```python
from build123d import *

# Parameters (mm, degrees)
STOCK_BATTERY_BASE_1_DEPTH   = 7.5
STOCK_BATTERY_BASE_1_2_DEPTH = 4.5
BOSS_EXTRUDE1_DEPTH          = 7.5
CUT_EXTRUDE1_DEPTH           = 7.5


# Read off the part's stored shape, not the designer's step: Stock-battery base-1
with BuildPart() as part:
    # Stock-battery base-1 outline → Stock-battery base-1 (new body)
    with BuildSketch(Plane.XY):
        with BuildLine():
            Line((32.459100066, 42.420690995), (16.459100066, 43.22938712))
            Line((16.459100066, 43.22938712), (16.459100066, -58.832087736))
            Line((16.459100066, -58.832087736), (113.496599029, -53.92747215))
            add(Edge.make_bspline(
                [(113.496599029, -53.92747215), (114.973875685, -53.76034768), (116.389465073, -53.408303088), (118.438931288, -52.658652366), (119.109837198, -52.372048444), (120.430638868, -51.735858399), (121.082915856, -51.384782434), (122.988929436, -50.267489711), (124.197203446, -49.437169981), (126.541735842, -47.677906536), (127.677620036, -46.748450374), (128.850515141, -45.74891878), (128.904828159, -45.702543351), (128.959100066, -45.656116492)],
                knots=[0, 0, 0, 0, 0.125, 0.125, 0.1875, 0.1875, 0.25, 0.25, 0.375, 0.375, 0.5, 0.5, 0.506074438, 0.506074438, 0.506074438, 0.506074438], degree=3))
            Line((128.959100066, -45.656116492), (133.959100066, -45.656116492))
            Line((133.959100066, -45.656116492), (133.959100066, 33.628624999))
            Line((133.959100066, 33.628624999), (128.959100066, 33.628624999))
            add(Edge.make_bspline(
                [(128.959100066, 33.628624999), (128.913387154, 33.667730585), (127.751192536, 34.660386778), (126.568806099, 35.629041088), (124.805320754, 36.953884089), (124.207009004, 37.38378621), (122.992052543, 38.206145046), (122.374602128, 38.599251589), (120.484333172, 39.709851881), (119.174169326, 40.359663675), (117.093195419, 41.124643977), (116.387101294, 41.341482025), (114.957490187, 41.687263925), (114.232477088, 41.816732683), (113.496599029, 41.899982649)],
                knots=[0.494878569, 0.494878569, 0.494878569, 0.494878569, 0.5, 0.625, 0.625, 0.6875, 0.6875, 0.75, 0.75, 0.875, 0.875, 0.9375, 0.9375, 1, 1, 1, 1], degree=3))
            Line((113.496599029, 41.899982649), (32.459100066, 45.99590211))
            Line((32.459100066, 45.99590211), (32.459100066, 42.420690995))
        make_face()
        Polygon((112.616329261, 31.931709487), (112.616012614, -43.959214992), (98.959100066, -44.649483258), (98.959100066, 32.621993758), align=None, mode=Mode.SUBTRACT)
    extrude(amount=STOCK_BATTERY_BASE_1_DEPTH)

    # Stock-battery base-1 2 outline → Stock-battery base-1 2 (add)
    with BuildSketch(Plane.XY):
        Polygon((32.459100066, 45.99590211), (16.459100066, 46.804598235), (16.459100066, 43.22938712), (32.459100066, 42.420690995), align=None)
    extrude(amount=STOCK_BATTERY_BASE_1_2_DEPTH)

    # Sketch1 → Boss-Extrude1 (add)
    with BuildSketch(Plane.ZY.offset(-16.459100066)):
        Polygon((0, 46.804598235), (0, -58.832087736), (7.5, -58.832087736), (7.5, 43.22938712), (4.5, 43.22938712), (4.5, 46.804598235), align=None)
    extrude(amount=BOSS_EXTRUDE1_DEPTH)

    # Sketch2 → Cut-Extrude1 (cut)
    with BuildSketch(Plane.ZY.offset(-8.959100066)):
        Polygon((2.7, 41.42938712), (1.8, 41.42938712), (1.8, -57.032087736), (5.7, -57.032087736), (5.7, 41.42938712), align=None)
    extrude(amount=-CUT_EXTRUDE1_DEPTH, mode=Mode.SUBTRACT)


solid = part.part
```
CAD build for the part. Positions are in the model's coordinates, mm. A direction names the side the tool comes from. Round coordinates to 2 decimals unless told otherwise and drop trailing zeros. Write each loop counter-clockwise with the first axis right and the second up, starting at its lowest first coordinate (ties: lowest second). Pieces come first, ordered by that corner, then holes. Notation, with made-up numbers: (33, -4.5) - (53, -4.5) arc R25 ccw to (53, 25.5) - close; hole circle Ø7 at (6, 46.5). An arc over 180 degrees is marked (long way). Return JSON: item names as keys, results as strings. Group by question number.
Item 1: Mould opens along X. For faces 4 (the face through (131, -45.656, 4)), 5 (the face through (105.69, 32.28, 3.7)), 6 (the face through (16.459, -7, 4)) say: +X half, -X half, draft (parallel to the pull), parting line (faces both ways), or undercut.
Item 2: 3-axis set-ups, long thin cutter, end or side, ignore diameter. For faces 1 (the face through (13, -8, 5.7)), 2 (the face through (131, 33.629, 4)), 3 (the face through (13, 43.229, 6)): which of +Z, -Z, +X, -X, +Y, -Y reach the whole face in a straight line?
Item 3: Band-saw the part on B-B on x = 102.5. List the corners of the cut face in (y, z).
Item 4: Probe probe 1 along X at (y, z) = (-17.5, 1.75); probe 2 along X at (y, z) = (-36, 4); probe 3 along Y at (x, z) = (105, 2.5). List the from-to ranges inside material, lowest first.
Item 5: Flat gauge pins, fed straight in: pin 1 Ø1.5 at (y, z) = (8, 4) entering from -X; pin 2 Ø6 at (x, y) = (108, -31.5) entering from +Z; pin 3 Ø1.5 at (x, z) = (132, 5) entering from +Y. Where does each tip first touch, or does it go through?
Item 6: Band-saw the part on A-A on y = -27.5. List the corners of the cut face in (x, z).
Item 7: Band-saw the part on D-D on x = 44.5. List the corners of the cut face in (y, z).
Resolved:
{
 "1": {"face 4": "draft", "face 5": "undercut", "face 6": "-X half"},
 "2": {"face 1": "-X", "face 2": "+Z, -Z, +X, +Y", "face 3": "+Z, -X, +Y"},
 "3": {"outline": "(-54.48, 0) - (-44.47, 0) - (-44.47, 7.5) - (-54.48, 7.5) - close; (32.44, 0) - (42.46, 0) - (42.46, 7.5) - (32.44, 7.5) - close"},
 "4": {"probe 1": "x = 8.96 to 98.96, 112.62 to 133.96", "probe 2": "x = 16.46 to 98.96, 112.62 to 133.96", "probe 3": "y = -54.36 to -44.34, 32.32 to 42.33"},
 "5": {"pin 1": "stops at x = 16.46", "pin 2": "passes through", "pin 3": "stops at y = 33.63"},
 "6": {"outline": "(8.96, 0) - (98.96, 0) - (98.96, 7.5) - (8.96, 7.5) - (8.96, 5.7) - (16.46, 5.7) - (16.46, 1.8) - (8.96, 1.8) - close; (112.62, 0) - (133.96, 0) - (133.96, 7.5) - (112.62, 7.5) - close"},
 "7": {"outline": "(-57.41, 0) - (45.39, 0) - (45.39, 7.5) - (-57.41, 7.5) - close"}
}
